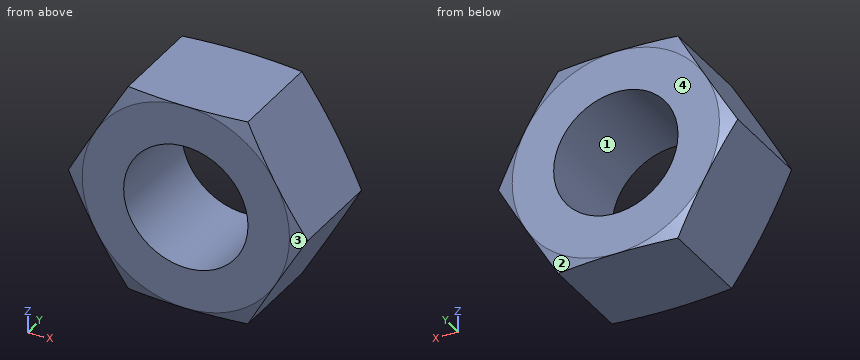
from build123d import *

# Parameters (mm, degrees)
SKETCH1_R           = 3
BOSS_EXTRUDE1_DEPTH = 5
SKETCH2_OUTSIDE_W   = 18.366
SKETCH2_OUTSIDE_H   = 16.818
SKETCH2_OUTSIDE_R   = 5
CUT_EXTRUDE2_DEPTH  = 0.2
CUT_EXTRUDE2_TAPER  = 76
SKETCH3_OUTSIDE_W   = 18.366
SKETCH3_OUTSIDE_H   = 16.818
SKETCH3_OUTSIDE_R   = 5
CUT_EXTRUDE3_DEPTH  = 0.2
CUT_EXTRUDE3_TAPER  = 76


with BuildPart() as part:
    # Sketch1 → Boss-Extrude1 (new body)
    with BuildSketch(Plane(origin=(0, 0, 0), x_dir=(1, 0, 0), z_dir=(0, 1, 0))):
        Polygon((5.773502692, 0), (2.886751346, 5), (-2.886751346, 5), (-5.773502692, 0), (-2.886751346, -5), (2.886751346, -5), align=None)
        Circle(SKETCH1_R, mode=Mode.SUBTRACT)
    extrude(amount=BOSS_EXTRUDE1_DEPTH)

    # Sketch2 outside → Cut-Extrude2 (cut)
    with BuildSketch(Plane(origin=(0, 5, 0), x_dir=(1, 0, 0), z_dir=(0, 1, 0))):
        Rectangle(SKETCH2_OUTSIDE_W, SKETCH2_OUTSIDE_H)
        Circle(SKETCH2_OUTSIDE_R, mode=Mode.SUBTRACT)
    extrude(amount=-CUT_EXTRUDE2_DEPTH, taper=CUT_EXTRUDE2_TAPER, mode=Mode.SUBTRACT)

    # Sketch3 outside → Cut-Extrude3 (cut)
    with BuildSketch(Plane.XZ):
        Rectangle(SKETCH3_OUTSIDE_W, SKETCH3_OUTSIDE_H)
        Circle(SKETCH3_OUTSIDE_R, mode=Mode.SUBTRACT)
    extrude(amount=-CUT_EXTRUDE3_DEPTH, taper=CUT_EXTRUDE3_TAPER, mode=Mode.SUBTRACT)


solid = part.part
Work out the finished part from the listing and answer in its coordinate system (mm). Face numbers are marked on the shaded views. Give positions to 0.01 mm unless a question says otherwise; leave off trailing zeros. Loops run counter-clockwise (first coordinate to the right, second up) from the corner with the lowest first, then second, coordinate; pieces in that order, holes last. Notation, with made-up numbers: (34, 24.25) -> (46, 24.25) arc R12 cw to (46, 28.25) -> close; hole circle Ø2 at (61, 72). An arc over 180 degrees is marked (long way). Use a Markdown table: item, result. Add a question column.
1. Determine the mould class of the marked faces 1, 2, 3 and 4 for opening direction Z: released by +Z, released by -Z, zero draft, split by the parting line, or undercut.
2. Flat-ended cylindrical pins translate along their axes: pin 1 Ø5 at (x, z) = (-1.5, 2.5) entering from -Y; pin 2 Ø3.5 at (x, z) = (0, 0) entering from +Y. Find the tip coordinate at first contact, or state that the pin passes through.
3. Find the intervals of material crossed by probe 1 along X at (y, z) = (2.7, 1.75); probe 2 along X at (y, z) = (1.5, 2); probe 3 along X at (y, z) = (4.4, -4), in increasing order.
4. Section A-A on y = 3.7 is taken. Determine the outline of the cut face in (x, z).
Results below:
| question | item | result |
|---|---|---|
| 1 | face 1 | undercut |
| 1 | face 2 | released by -Z |
| 1 | face 3 | split by the parting line |
| 1 | face 4 | zero draft |
| 2 | pin 1 | stops at y = 0 |
| 2 | pin 2 | passes through |
| 3 | probe 1 | x = -4.76 to -2.44, 2.44 to 4.76 |
| 3 | probe 2 | x = -4.62 to -2.24, 2.24 to 4.62 |
| 3 | probe 3 | x = -3.46 to 3.46 |
| 4 | outline | (-5.77, 0) -> (-2.89, -5) -> (2.89, -5) -> (5.77, 0) -> (2.89, 5) -> (-2.89, 5) -> close; hole circle Ø6 at (0, 0) |
